Here's how the part is built. I have some questions about the finished solid (model axes, mm). Face numbers are marked on the shaded views. A direction names the side the tool comes from. Round coordinates to 2 decimals unless told otherwise and drop trailing zeros. Write each loop counter-clockwise with the first axis right and the second up, starting at its lowest first coordinate (ties: lowest second). Pieces come first, ordered by that corner, then holes. Notation, with made-up numbers: (48, -0.5) - (76, -0.5) arc R16 cw to (76, 7.5) - close; hole circle Ø10 at (-13, 81). An arc over 180 degrees is marked (long way). One line per question, with ' | ' between items. Start each with the question number.
(1) Will this pin go through, and if not, where does the flat tip stop? pin 1 (2 mm diameter, centred on y = 4.5, z = 1, fed in from +X) (3 decimals).
(2) For the marked faces 1 and 2, which set-ups out of +Z, -Z, +X, -X, +Y, -Y let a thin tool reach every point of the face, with its end or its side?
(3) Imagine slicing it at C-C (z = 3.25). Write out the boundary of the cut face in (x, y), plus the area to 3 significant figures.
(4) If I drill on L1, parallel to Z at x = -7.5, y = -7.25; L2, parallel to X at y = -0.25, z = 3.05; L3, parallel to X at y = -13.5, z = 1.75, over which ranges is the centre line in solid material (lowest first)?
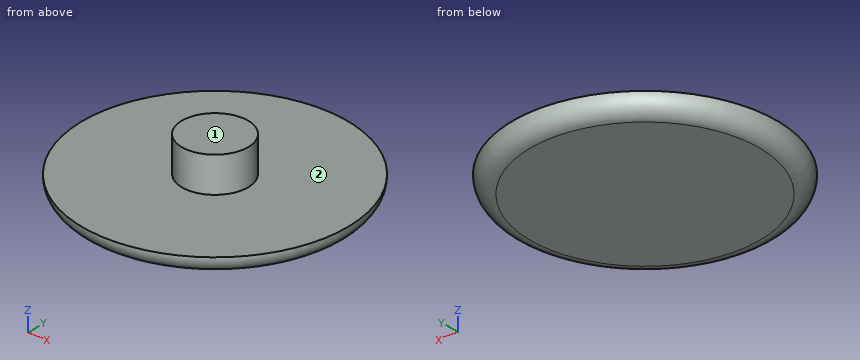
from build123d import *

# Parameters (mm, degrees)
F0_R     = 15
F0_R_2   = 3.75
F1_DEPTH = 2
F2_R     = 3.75
F3_DEPTH = 4
F4_R     = 1.99999


# Not quite as in the source:
# - a fillet or chamfer is up to 0.001 mm smaller than in the source, because OpenCascade refuses the exact size


with BuildPart() as f1:
    # F0 (on Top) → F1 (new body)
    with BuildSketch(Plane.XY):
        Circle(F0_R)
        Circle(F0_R_2, mode=Mode.SUBTRACT)
        Circle(F0_R_2)
    extrude(amount=F1_DEPTH)

    # F2 (on face) → F3 (join)
    with BuildSketch(Plane.XY.offset(2)):
        Circle(F2_R)
    extrude(amount=F3_DEPTH)

    # F4 (radius 2 in the source; OpenCascade refuses exactly that, so slightly less here)
    f4_edges = [f1.edges().sort_by_distance(p)[0] for p in [
        (-15, 0, 0),
    ]]
    fillet(f4_edges, radius=F4_R)


solid = f1.part
Check sheet entries:
1) pin 1: x = 14.495
2) face 1: +Z, +X, -X, +Y, -Y | face 2: +Z
3) outline: circle Ø7.5 at (0, 0) | area: 44.2 mm^2
4) L1: 0 to 2 | L2: -3.74 to 3.74 | L3: -6.5 to 6.5
